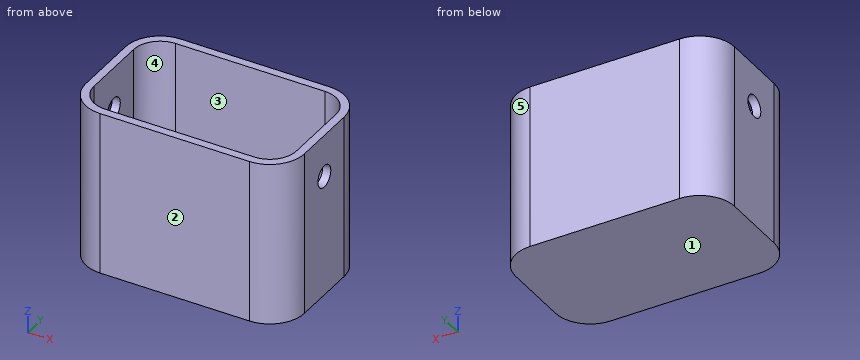
from build123d import *

# Parameters (mm, degrees)
F0_W     = 80
F0_H     = 50
F1_DEPTH = 60
F2_R     = 12.7
F3_T     = -3
F5_D     = 8


# Not quite as in the source:
# - a feature names something its author has since deleted; it is built from what else it names


with BuildPart() as f1:
    # F0 (on Top) → F1 (new body)
    with BuildSketch(Plane.XY):
        with Locations((-2.1280694621, 0)):
            Rectangle(F0_W, F0_H)
    extrude(amount=F1_DEPTH)

    # F2
    f2_edges = [f1.edges().sort_by_distance(p)[0] for p in [
        (-42.128069, -25, 30),
        (37.871931, 25, 30),
        (37.871931, -25, 30),
        (-42.128069, 25, 30),
    ]]
    fillet(f2_edges, radius=F2_R)

    # F3
    f3_openings = [f1.faces().sort_by_distance(p)[0] for p in [
        (-2.128069, 0, 60),
    ]]
    offset(amount=F3_T, openings=f3_openings)

    # F5 (through all)
    with Locations(Plane.YZ.offset(37.8719305379)):
        with Locations((0, 44.5649288595)):
            Hole(F5_D / 2)


solid = f1.part
Read the model definition and answer for the solid it produces. Units are mm, in the model's axes. Face numbers are marked on the shaded views. A direction names the side the tool comes from. Round coordinates to 2 decimals unless told otherwise and drop trailing zeros. Loops run counter-clockwise (first coordinate to the right, second up) from the corner with the lowest first, then second, coordinate; pieces in that order, holes last.
Q1. Section D-D on y = -7.5 is taken. Write down the section's boundary in (x, z), and give its area (3 significant figures).
Q2. Section C-C on x = -0.5 is taken. Write down the section's boundary in (y, z).
Q3. Consider probe 1 along X at (y, z) = (7.5, 8.5); probe 2 along Z at (x, y) = (-41.4, 0); probe 3 along Y at (x, z) = (-19.5, 51). Determine where each line is inside the solid, lowest interval first.
Q4. Determine the mould class of the marked faces 1, 2 and 3 for opening direction Y: released by +Y, released by -Y, zero draft, split by the parting line, or undercut.
Q5. Section A-A on y = 0 is taken. Write down the section's boundary in (x, z), and give its area (3 significant figures).
Q6. Which of the six approach directions +Z, -Z, +X, -X, +Y, -Y give full straight-line access (tool end or side, diameter ignored) to the marked faces 4 and 5?
Q7. Section B-B on z = 22 is taken. Write down the section's boundary in (x, y), and give its area (3 significant figures).
Q8. Each of these flat-tipped pins is pushed along its axis until it touches: pin 1 (2 mm diameter, centred on x = 13, y = 3, fed in from -Z); pin 2 (4 mm diameter, centred on x = 10, y = -10.5, fed in from +Z); pin 3 (7 mm diameter, centred on y = 0, z = 44.56, fed in from +X); pin 4 (8 mm diameter, centred on y = -18.5, z = 45.5, fed in from -X). Where does it stop, or does it pass through?
Output:
1. outline: (-42.13, 0) - (37.87, 0) - (37.87, 60) - (34.87, 60) - (34.87, 3) - (-39.13, 3) - (-39.13, 60) - (-42.13, 60) - close
1. area: 582 mm2
2. outline: (-25, 0) - (25, 0) - (25, 60) - (22, 60) - (22, 3) - (-22, 3) - (-22, 60) - (-25, 60) - close
3. probe 1: x = -42.13 to -39.13, 34.87 to 37.87
3. probe 2: z = 0 to 40.56, 48.56 to 60
3. probe 3: y = -25 to -22, 22 to 25
4. face 1: zero draft
4. face 2: released by -Y
4. face 3: undercut
5. outline: (-42.13, 0) - (37.87, 0) - (37.87, 40.56) - (34.87, 40.56) - (34.87, 3) - (-39.13, 3) - (-39.13, 40.56) - (-42.13, 40.56) - close; (-42.13, 48.56) - (-39.13, 48.56) - (-39.13, 60) - (-42.13, 60) - close; (34.87, 48.56) - (37.87, 48.56) - (37.87, 60) - (34.87, 60) - close
5. area: 534 mm2
6. face 4: +Z
6. face 5: +Z, -Z, +X, +Y
7. outline: (-42.13, -12.3) arc R12.7 ccw to (-29.43, -25) - (25.17, -25) arc R12.7 ccw to (37.87, -12.3) - (37.87, 12.3) arc R12.7 ccw to (25.17, 25) - (-29.43, 25) arc R12.7 ccw to (-42.13, 12.3) - close; hole (-39.13, -12.3) arc R9.7 ccw to (-29.43, -22) - (25.17, -22) arc R9.7 ccw to (34.87, -12.3) - (34.87, 12.3) arc R9.7 ccw to (25.17, 22) - (-29.43, 22) arc R9.7 ccw to (-39.13, 12.3) - close
7. area: 686 mm2
8. pin 1: stops at z = 0
8. pin 2: stops at z = 3
8. pin 3: passes through
8. pin 4: stops at x = -41.94
